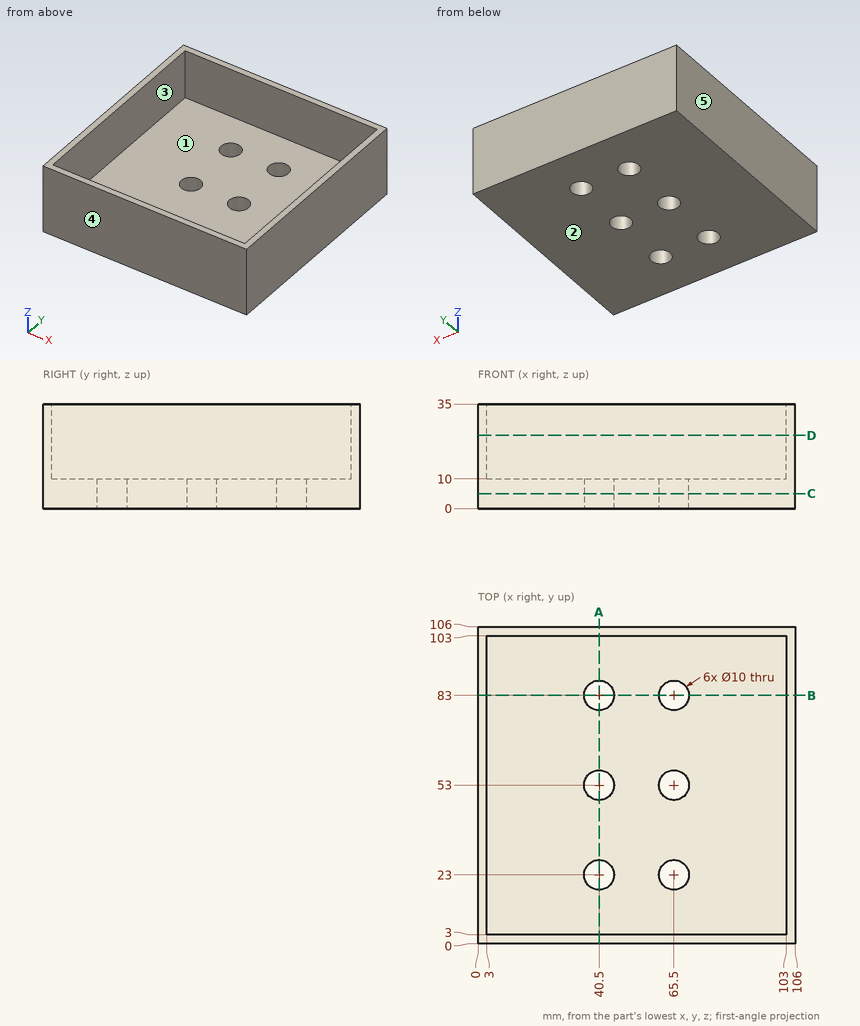
Design review of the part shown in the three views and the two pictorial views. Dimensions are in mm from the part's minimum x, y and z. A direction names the side the tool comes from. Round coordinates to 2 decimals unless told otherwise and drop trailing zeros. Loops run counter-clockwise (first coordinate to the right, second up) from the corner with the lowest first, then second, coordinate; pieces in that order, holes last. Notation, with made-up numbers: (28.5, 59) -> (84.5, 59) arc R10 cw to (84.5, 75) -> close; hole circle Ø7 at (68, 8.25). An arc over 180 degrees is marked (long way). Return JSON: item names as keys, results as strings.
(1) For line 1 (X direction, y = 83, z = 4.5); line 2 (Y direction, x = 65.5, z = 3); line 3 (X direction, y = 24.5, z = 15), list the stretches that pass through material, from the lowest coordinate up.
Solved:
{"line 1": "0 to 35.5, 45.5 to 60.5, 70.5 to 106", "line 2": "0 to 18, 28 to 48, 58 to 78, 88 to 106", "line 3": "0 to 3, 103 to 106"}
(2) Add section D-D on z = 24.5. Write out the cut boundary in (x, y), plus the area to 3 significant figures.
Solved:
{"outline": "(0, 0) -> (106, 0) -> (106, 106) -> (0, 106) -> close; hole (3, 3) -> (103, 3) -> (103, 103) -> (3, 103) -> close", "area": "1,240 mm2"}
(3) Add section B-B on y = 83. Write out the cut boundary in (x, z).
Solved:
{"outline": "(0, 0) -> (35.5, 0) -> (35.5, 10) -> (3, 10) -> (3, 35) -> (0, 35) -> close; (45.5, 0) -> (60.5, 0) -> (60.5, 10) -> (45.5, 10) -> close; (70.5, 0) -> (106, 0) -> (106, 35) -> (103, 35) -> (103, 10) -> (70.5, 10) -> close"}
(4) For the marked faces 1 and 2, list the 3-axis set-ups (+Z, -Z, +X, -X, +Y, -Y) from which the entire face can be reached by the end or side of a thin tool; tool diameter is ignored.
Solved:
{"face 1": "+Z", "face 2": "-Z, +X, -X, +Y, -Y"}
(5) Add section C-C on z = 5. Write out the cut boundary in (x, y), plus the area to 3 significant figures.
Solved:
{"outline": "(0, 0) -> (106, 0) -> (106, 106) -> (0, 106) -> close; hole circle Ø10 at (40.5, 23); hole circle Ø10 at (40.5, 53); hole circle Ø10 at (40.5, 83); hole circle Ø10 at (65.5, 23); hole circle Ø10 at (65.5, 53); hole circle Ø10 at (65.5, 83)", "area": "10,800 mm2"}
(6) For pin 1 (11.5 mm diameter, centred on x = 40.5, y = 83, fed in from +Z); pin 2 (8 mm diameter, centred on x = 65.5, y = 23, fed in from +Z), all flat-tipped, find the tip position at first contact; note any pin that passes through.
Solved:
{"pin 1": "z = 10", "pin 2": "through"}
(7) The part is to be moulded in two halves that separate along Y. For the marked faces 3, 4 and 5, say which applies: released by +Y, released by -Y, zero draft, split by the parting line, or undercut.
Solved:
{"face 3": "undercut", "face 4": "released by -Y", "face 5": "zero draft"}
(8) Add section A-A on x = 40.5. Write out the cut boundary in (y, z), plus the area to 3 significant figures.
Solved:
{"outline": "(0, 0) -> (18, 0) -> (18, 10) -> (3, 10) -> (3, 35) -> (0, 35) -> close; (28, 0) -> (48, 0) -> (48, 10) -> (28, 10) -> close; (58, 0) -> (78, 0) -> (78, 10) -> (58, 10) -> close; (88, 0) -> (106, 0) -> (106, 35) -> (103, 35) -> (103, 10) -> (88, 10) -> close", "area": "910 mm2"}
